Design review of the part built by this model. Coordinates are the model's own, in mm. A direction names the side the tool comes from. Coordinates: 2 decimals unless noted, no trailing zeros. Loops run counter-clockwise (first coordinate to the right, second up) from the corner with the lowest first, then second, coordinate; pieces in that order, holes last. Notation, with made-up numbers: (37.5, 18) -> (60.5, 18) arc R19 ccw to (60.5, 37) -> close; hole circle Ø5 at (19.25, 30). An arc over 180 degrees is marked (long way). Answer as a JSON object with one key per item and string values.
```python
from build123d import *

# Parameters (mm, degrees)
F1_DEPTH = 63.5
F2_DEPTH = 25.4
F0_W     = 25.4
F0_H     = 19.05
F3_DEPTH = 25.4
F4_DEPTH = 7.9375
F6_R     = 6.35


with BuildPart() as f1:
    # F0 (on Front) → F1 (new body, symmetric)
    with BuildSketch(Plane.XZ):
        Polygon((22.225, 9.525), (-41.275, 9.525), (-41.275, -9.525), (41.275, -9.525), (41.275, 9.525), align=None)
    extrude(amount=F1_DEPTH, both=True)

    # F0 (on Front) → F2 (join, symmetric)
    with BuildSketch(Plane.XZ):
        with BuildLine():
            Line((22.225, 27.0002), (22.225, 9.525))
            Line((22.225, 9.525), (41.275, 9.525))
            Line((41.275, 9.525), (41.275, 27.0002))
            ThreePointArc((41.275, 27.0002), (45.9246798487, 38.2255201513), (57.15, 42.8752))
            Line((57.15, 42.8752), (60.325, 42.8752))
            Line((60.325, 42.8752), (60.325, 61.9252))
            Line((60.325, 61.9252), (57.15, 61.9252))
            ThreePointArc((57.15, 61.9252), (32.4542956671, 51.6959043329), (22.225, 27.0002))
        make_face()
    extrude(amount=F2_DEPTH, both=True)

    # F0 (on Front) → F3 (join, symmetric)
    with BuildSketch(Plane.XZ):
        with Locations((73.025, 52.4002)):
            Rectangle(F0_W, F0_H)
    extrude(amount=F3_DEPTH, both=True)

    # F0 (on Front) → F4 (join, symmetric)
    with BuildSketch(Plane.XZ):
        with BuildLine():
            add(Edge.make_bspline(
                [(-41.275, 9.525), (-40.1356369257, 51.84443295), (0, 62.6272857189), (57.15, 61.9252)],
                knots=[0, 0, 0, 0, 111.5045361635, 111.5045361635, 111.5045361635, 111.5045361635], degree=3))
            Line((-41.275, 9.525), (22.225, 9.525))
            Line((22.225, 9.525), (22.225, 27.0002))
            ThreePointArc((22.225, 27.0002), (32.4542956671, 51.6959043329), (57.15, 61.9252))
        make_face()
    extrude(amount=F4_DEPTH, both=True)

    # F0 (on Front) → F5 (revolve)
    with BuildSketch(Plane.XZ):
        Polygon((85.725, 66.675), (85.725, 61.9252), (85.725, 42.8752), (85.725, 38.1), (111.125, 38.1), (111.125, 66.675), align=None)
    revolve(axis=Axis((85.725, 0, 52.3875), (0, 0, 1)))

    # F6
    f6_edges = [f1.edges().sort_by_distance(p)[0] for p in [
        (41.275, -63.5, 0),
        (-41.275, -63.5, 0),
        (41.275, 63.5, 0),
        (-41.275, 63.5, 0),
    ]]
    fillet(f6_edges, radius=F6_R)


solid = f1.part
```
1) For faces 1 (the cylindrical face through (32.73, -16.79, 51.97)), 2 (the cylindrical face through (32.73, 16.55, 51.97)), 3 (the flat face through (46, -25.4, 42)), 4 (the flat face through (60, 2, 42.875)), 5 (the flat face through (41.275, -1, 4)), list the 3-axis set-ups (+Z, -Z, +X, -X, +Y, -Y) from which the entire face can be reached by the end or side of a thin tool; tool diameter is ignored.
Completed:
{"face 1": "+Z, -X, -Y", "face 2": "+Z, -X, +Y", "face 3": "+Z, +X, -X, -Y", "face 4": "-Z", "face 5": "-Z, +X, +Y, -Y"}
2) Clearance check with flat-ended pins moving along their axes: pin 1 Ø12 at (x, y) = (11.5, -4) entering from +Z; pin 2 Ø2 at (x, y) = (87, 27.5) entering from -Z; pin 3 Ø10 at (x, z) = (42, 15) entering from +Y; pin 4 Ø8.5 at (x, y) = (76.5, -10.5) entering from -Z. State where each tip first meets the part, or that it passes through.
Completed:
{"pin 1": "z = 59.94", "pin 2": "through", "pin 3": "y = 25.4", "pin 4": "z = 38.1"}
3) The part is to be moulded in two halves that separate along X. For faces 6 (the flat face through (22.225, 17, 18)), 7 (the cylindrical face through (45.8, -0.4, 38.1)), 8 (the flat face through (1, -36, 9.525)), say which applies: pulls with the +X half, pulls with the -X half, needs draft (parallel to the pull), parting line crosses it, or undercut.
Completed:
{"face 6": "pulls with the -X half", "face 7": "undercut", "face 8": "needs draft"}
4) Add section A-A, the plane z = -3. Give the boundary of the cut face in (x, y) (3 decimals), and give its area (3 significant figures).
Completed:
{"outline": "(-41.275, -57.15) arc R6.35 ccw to (-34.925, -63.5) -> (34.925, -63.5) arc R6.35 ccw to (41.275, -57.15) -> (41.275, 57.15) arc R6.35 ccw to (34.925, 63.5) -> (-34.925, 63.5) arc R6.35 ccw to (-41.275, 57.15) -> close", "area": "10,400 mm²"}
5) Add section B-B, the plane y = 19. Give the boundary of the cut face in (x, z) (3 decimals), and give its area (3 significant figures).
Completed:
{"outline": "(-41.275, -9.525) -> (41.275, -9.525) -> (41.275, 27) arc R15.875 cw to (57.15, 42.875) -> (68.868, 42.875) -> (68.868, 38.1) -> (102.582, 38.1) -> (102.582, 66.675) -> (68.868, 66.675) -> (68.868, 61.925) -> (57.15, 61.925) arc R34.925 ccw to (22.225, 27) -> (22.225, 9.525) -> (-41.275, 9.525) -> close", "area": "3,850 mm²"}
6) Add section C-C, the plane y = -48.5. Give the boundary of the cut face in (x, z) (3 decimals), and give its area (3 significant figures).
Completed:
{"outline": "(-41.275, -9.525) -> (41.275, -9.525) -> (41.275, 9.525) -> (-41.275, 9.525) -> close", "area": "1,570 mm²"}
7) Wall thickness on probe 1 along Y at (x, z) = (50.5, 61.5); probe 2 along Z at (x, y) = (-20, -40) (3 decimals); probe 3 along X at (y, z) = (-29, 1.5) (3 decimals): over which ranges is each line inside the solid? List them lowest first.
Completed:
{"probe 1": "-7.94 to 7.94", "probe 2": "-9.525 to 9.525", "probe 3": "-41.275 to 41.275"}
